from build123d import *

# Parameters (mm, degrees)
SKETCH1_R           = 15
BOSS_EXTRUDE1_DEPTH = 2
SKETCH2_R           = 3.58
SKETCH2_R_2         = 2.58
BOSS_EXTRUDE2_DEPTH = 55
SKETCH3_R           = 2.58
CUT_EXTRUDE1_DEPTH  = 55


with BuildPart() as part:
    # Sketch1 → Boss-Extrude1 (new body)
    with BuildSketch(Plane.XY):
        Circle(SKETCH1_R)
    extrude(amount=BOSS_EXTRUDE1_DEPTH)

    # Sketch2 → Boss-Extrude2 (add)
    with BuildSketch(Plane.XY.offset(2)):
        Circle(SKETCH2_R)
        Circle(SKETCH2_R_2, mode=Mode.SUBTRACT)
    extrude(amount=BOSS_EXTRUDE2_DEPTH)

    # Sketch3 → Cut-Extrude1 (cut)
    with BuildSketch(Plane.XY.offset(2)):
        Circle(SKETCH3_R)
    extrude(amount=-CUT_EXTRUDE1_DEPTH, mode=Mode.SUBTRACT)


solid = part.part
Model file for the job. Use its own axes, mm. A direction names the side the tool comes from. Coordinates: 2 decimals unless noted, no trailing zeros. Order: outer loops, then holes, each group sorted by start corner. A loop starts at its lowest first (then second) coordinate and runs counter-clockwise, first axis right, second up. Notation, with made-up numbers: M 28,19.25 L 38,19.25 A12 ccw 38,35.25 Z; hole C -3,34 d9. An arc over 180 degrees is marked long. Return JSON: item names as keys, results as strings.
1. Saw through at A-A (y = 0). Give the cut face in (x, z).
Ans:
{"outline": "M -15,0 L -2.58,0 L -2.58,57 L -3.58,57 L -3.58,2 L -15,2 Z; M 2.58,0 L 15,0 L 15,2 L 3.58,2 L 3.58,57 L 2.58,57 Z"}
2. Tool access for faces 1 (the face through (-0.776, -3.495, 29.115)), 2 (the face through (2, 2, 57)): list every direction of +Z, -Z, +X, -X, +Y, -Y with a clear straight run to the whole face (end or side of a thin tool).
Ans:
{"face 1": "+Z", "face 2": "+Z, +X, -X, +Y, -Y"}
3. Saw through at D-D (y = -11.5). Give the cut face in (x, z).
Ans:
{"outline": "M -9.63,0 L 9.63,0 L 9.63,2 L -9.63,2 Z"}
4. Flat gauge pins, fed straight in: pin 1 (2 mm diameter, centred on x = 4, y = 7, fed in from +Z); pin 2 (6 mm diameter, centred on y = -3.5, z = 15.5, fed in from -X); pin 3 (2 mm diameter, centred on y = -1.5, z = 33.5, fed in from +X); pin 4 (3 mm diameter, centred on x = -2.5, y = -7.5, fed in from -Z). Where does each tip first touch, or does it go through?
Ans:
{"pin 1": "z = 2", "pin 2": "x = -3.54", "pin 3": "x = 3.54", "pin 4": "z = 0"}
5. Saw through at C-C (z = 29). Give the cut face in (x, y), and give its area (3 significant figures).
Ans:
{"outline": "C 0,0 d7.16; hole C 0,0 d5.16", "area": "19.4 mm^2"}
6. Drill centre lines: probe 1 along Y at (x, z) = (0, 45); probe 2 along Z at (x, y) = (-11.5, -9.5); probe 3 along Y at (x, z) = (0, 0.55). Where is each one in solid material? Low to high.
Ans:
{"probe 1": "-3.58 to -2.58, 2.58 to 3.58", "probe 2": "0 to 2", "probe 3": "-15 to -2.58, 2.58 to 15"}
